Print and shaded views of the part. All mm, measured from the part's lowest x, y and z. A direction names the side the tool comes from. Round coordinates to 2 decimals unless told otherwise and drop trailing zeros. Loops run counter-clockwise (first coordinate to the right, second up) from the corner with the lowest first, then second, coordinate; pieces in that order, holes last. Notation, with made-up numbers: (11.25, 53) - (32.25, 53) arc R27 ccw to (32.25, 90) - close; hole circle Ø10 at (69.5, 16.25). An arc over 180 degrees is marked (long way). Use one line per item in the form item = value. Start each with the question number.
Q1. Mould opens along Z. For the marked faces 3, 4 and 5 say: released by +Z, released by -Z, zero draft, split by the parting line, or undercut.
Q2. Drill centre lines: line 1 (Z direction, x = 5.5, y = 18) (1 decimal); line 2 (Z direction, x = 8.5, y = 13.5) (1 decimal); line 3 (Y direction, x = 16.5, z = 7.5). Where is each one in solid material? Low to high.
Q3. Saw through at A-A (y = 25.4). Give the cut face in (x, z), then the cut area to 3 significant figures.
Q4. Pin check, flat tips, straight feed: pin 1 (1.5 mm diameter, centred on x = 30, z = 18, fed in from -Y); pin 2 (2 mm diameter, centred on x = 42.5, z = 66, fed in from +Y) (1 decimal); pin 3 (2 mm diameter, centred on x = 11, z = 55.5, fed in from +Y). Stop position of each tip, or through.
Q5. Saw through at D-D (z = 70). Give the cut face in (x, y).
Q6. Saw through at C-C (z = 25). Give the cut face in (x, y).
Q7. 3-axis set-ups, long thin cutter, end or side, ignore diameter. For the marked faces 1 and 2: which of +Z, -Z, +X, -X, +Y, -Y reach the whole face in a straight line?
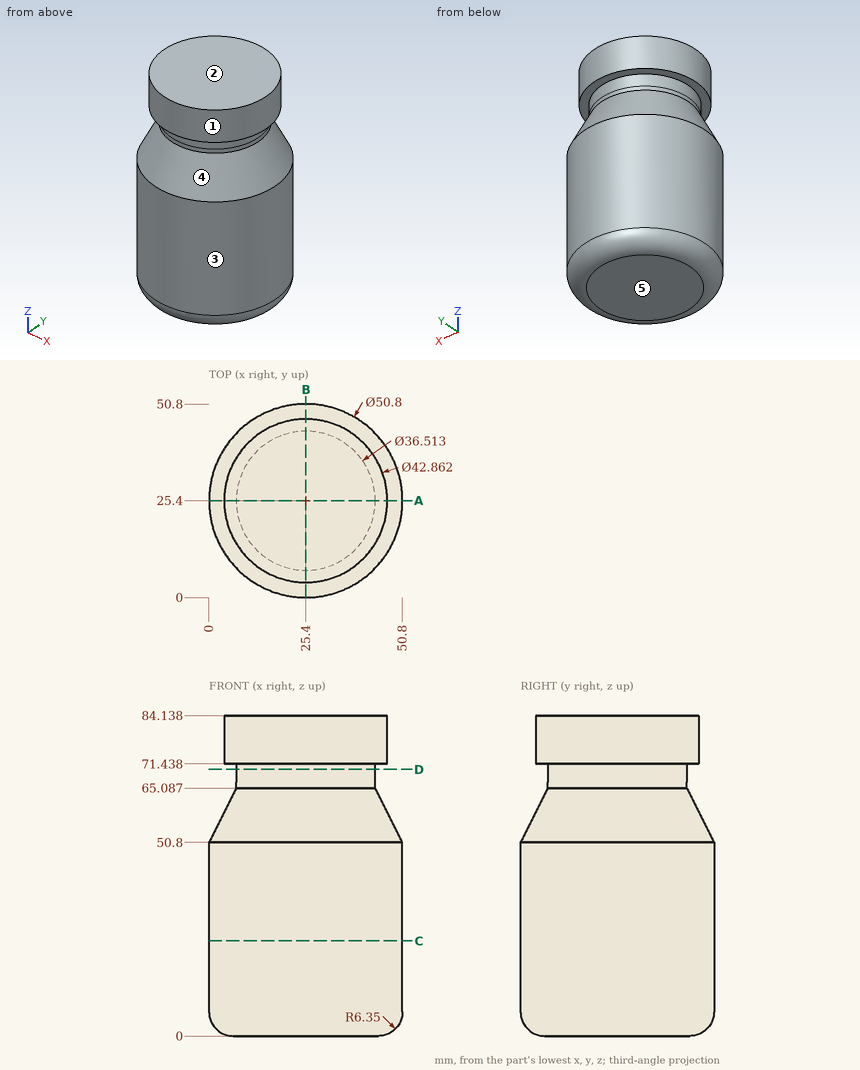
Report:
q1.face_3 = zero draft
q1.face_4 = undercut
q1.face_5 = released by -Z
q2.line_1 = 0.4 to 59.1, 71.4 to 84.1
q2.line_2 = 0.2 to 60.3, 71.4 to 84.1
q2.line_3 = 1.61 to 49.19
q3.outline = (0, 6.35) arc R6.35 ccw to (6.35, 0) - (44.45, 0) arc R6.35 ccw to (50.8, 6.35) - (50.8, 50.8) - (43.66, 65.09) - (43.66, 71.44) - (46.83, 71.44) - (46.83, 84.14) - (3.97, 84.14) - (3.97, 71.44) - (7.14, 71.44) - (7.14, 65.09) - (0, 50.8) - close
q3.area = 3,960 mm²
q4.pin_1 = 0.29
q4.pin_2 = 34
q4.pin_3 = 44.38
q5.outline = circle Ø36.51 at (25.4, 25.4)
q6.outline = circle Ø50.8 at (25.4, 25.4)
q7.face_1 = +Z
q7.face_2 = +Z, +X, -X, +Y, -Y
